Build history of the part. All positions in model axes, mm. Round coordinates to 2 decimals unless told otherwise and drop trailing zeros. Loops run counter-clockwise (first coordinate to the right, second up) from the corner with the lowest first, then second, coordinate; pieces in that order, holes last.
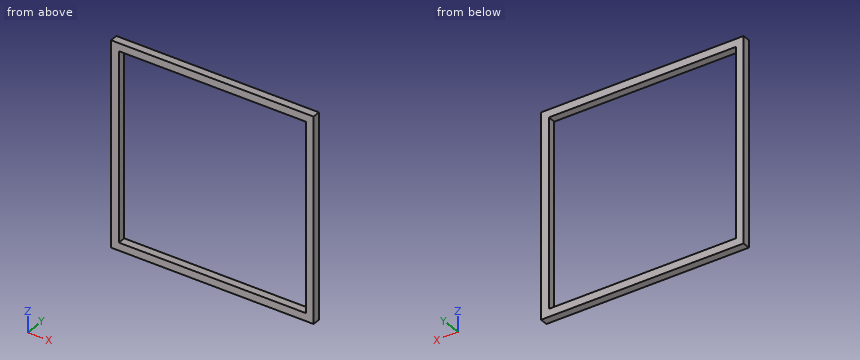
Autodesk Inventor part; units mm, degrees
ref_plane "YZ Plane" through (0, 0, 0) normal (1, 0, 0) x (0, 1, 0)
ref_plane "XZ Plane" through (0, 0, 0) normal (0, 1, 0) x (-1, 0, 0)
ref_plane "XY Plane" through (0, 0, 0) normal (0, 0, 1) x (1, 0, 0)
sketch "Sketch1" plane through (0, 0, 0) normal (0, 1, 0) x (-1, 0, 0)
  line L0 (8.7651, 9.9871) -> (-651.6349, 9.9871)
  line L1 (-651.6349, 9.9871) -> (-651.6349, -650.4129)
  line L2 (-651.6349, -650.4129) -> (8.7651, -650.4129)
  line L3 (8.7651, -650.4129) -> (8.7651, 9.9871)
  line L4 (-16.6349, -15.4129) -> (-626.2349, -15.4129)
  line L5 (-626.2349, -15.4129) -> (-626.2349, -625.0129)
  line L6 (-626.2349, -625.0129) -> (-16.6349, -625.0129)
  line L7 (-16.6349, -625.0129) -> (-16.6349, -15.4129)
  point P0 (0, 0)
  dimension "d0" = 660.4
  dimension "d1" = 660.4
  dimension "d2" = 25.4
sketch "Sketch2" plane through (0, 0, 0) normal (0, 1, 0) x (-1, 0, 0)
  line L0 (-333.5663, -626.2819) -> (-333.5663, -550.0819) construction
  line L1 (-625.3108, -550.0819) -> (-18.6287, -550.0819) construction
  point P0 (0, 0)
  dimension "d3" = 76.2
extrude "Extrusion1" add sketch "Sketch1" along normal blind 25.4
properties part number "Frame Outline"
(1) Probe line 1 (X direction, y = 4.25, z = -498.5); line 2 (Z direction, x = 495.5, y = 2). List the from-to ranges inside material, lowest first.
Responses:
line 1: x = -8.77 to 16.63, 626.23 to 651.63
line 2: z = -650.41 to -625.01, -15.41 to 9.99
(2) Slice it at B-B on x = 209. List the corners of the cut face in (y, z).
Responses:
outline: (0, -650.41) - (25.4, -650.41) - (25.4, -625.01) - (0, -625.01) - close; (0, -15.41) - (25.4, -15.41) - (25.4, 9.99) - (0, 9.99) - close
(3) Slice it at C-C on y = 14.25. List the corners of the cut face in (x, z), plus the area to 3 significant figures.
Responses:
outline: (-8.77, -650.41) - (651.63, -650.41) - (651.63, 9.99) - (-8.77, 9.99) - close; hole (16.63, -625.01) - (626.23, -625.01) - (626.23, -15.41) - (16.63, -15.41) - close
area: 64,500 mm2
(4) Slice it at A-A on z = -36. List the corners of the cut face in (x, y).
Responses:
outline: (-8.77, 0) - (16.63, 0) - (16.63, 25.4) - (-8.77, 25.4) - close; (626.23, 0) - (651.63, 0) - (651.63, 25.4) - (626.23, 25.4) - close
